from build123d import *

# Parameters (mm, degrees)
SKETCH2_R           = 4.5
BOSS_EXTRUDE1_DEPTH = 15
SKETCH4_R           = 4
CUT_EXTRUDE2_DEPTH  = 1.5
SKETCH5_R           = 3
CUT_EXTRUDE3_DEPTH  = 2.5
CUT_EXTRUDE4_DEPTH  = 6
SKETCH7_W           = 18
SKETCH7_H           = 2.5
BOSS_EXTRUDE2_DEPTH = 5


with BuildPart() as part:
    # Sketch2 → Boss-Extrude1 (new body)
    with BuildSketch(Plane(origin=(0, 0, 0), x_dir=(1, 0, 0), z_dir=(0, 1, 0))):
        Circle(SKETCH2_R)
    extrude(amount=BOSS_EXTRUDE1_DEPTH)

    # Sketch4 → Cut-Extrude2 (cut)
    with BuildSketch(Plane.XZ):
        with Locations((0, 0.009200476)):
            Circle(SKETCH4_R)
    extrude(amount=-CUT_EXTRUDE2_DEPTH, mode=Mode.SUBTRACT)

    # Sketch5 → Cut-Extrude3 (cut)
    with BuildSketch(Plane.XZ.offset(-1.5)):
        with Locations((0.006133651, -0.009200476)):
            Circle(SKETCH5_R)
    extrude(amount=-CUT_EXTRUDE3_DEPTH, mode=Mode.SUBTRACT)

    # Sketch6 → Cut-Extrude4 (cut)
    with BuildSketch(Plane.XZ.offset(-4)):
        with BuildLine():
            Line((-2.446188527, -1.739471433), (2.441510318, -1.739471433))
            ThreePointArc((2.441510318, -1.739471433), (2.997660896, 0.000528567), (2.441510318, 1.740528567))
            Line((2.441510318, 1.740528567), (-2.446188527, 1.740528567))
            ThreePointArc((-2.446188527, 1.740528567), (-3.002339104, 0.000528567), (-2.446188527, -1.739471433))
        make_face()
    extrude(amount=-CUT_EXTRUDE4_DEPTH, mode=Mode.SUBTRACT)

    # Sketch7 → Boss-Extrude2 (add)
    with BuildSketch(Plane(origin=(0, 15, 0), x_dir=(1, 0, 0), z_dir=(0, 1, 0))):
        Rectangle(SKETCH7_W, SKETCH7_H)
    extrude(amount=-BOSS_EXTRUDE2_DEPTH)


solid = part.part
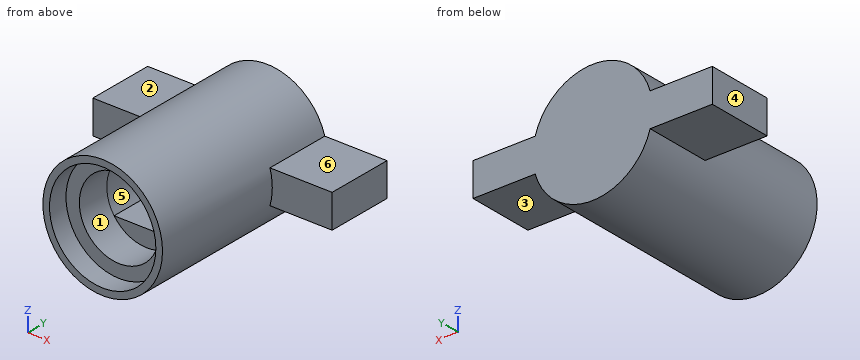
Work out the finished part from the listing and answer in its coordinate system (mm). Face numbers are marked on the shaded views. A direction names the side the tool comes from. Give positions to 0.01 mm unless a question says otherwise; leave off trailing zeros. Write each loop counter-clockwise with the first axis right and the second up, starting at its lowest first coordinate (ties: lowest second). Pieces come first, ordered by that corner, then holes. Notation, with made-up numbers: (73, 32) - (110, 32) arc R18 cw to (110, 54) - close; hole circle Ø9 at (28, 88.5). An arc over 180 degrees is marked (long way). One line per item, written item: value. Start each with the question number.
1. Consider probe 1 along Z at (x, y) = (0, 1.2); probe 2 along Y at (x, z) = (2.5, 3); probe 3 along Y at (x, z) = (5.25, 0). Determine where each line is inside the solid, lowest interval first.
2. Given pin 1 (2.5 mm diameter, centred on x = -2, z = 1.5, fed in from -Y); pin 2 (1.5 mm diameter, centred on x = 1, y = 7, fed in from -Z); pin 3 (5 mm diameter, centred on x = -6.5, y = 11.5, fed in from -Z), each flat-ended and moving along its own axis, determine where each tip first touches the part or whether it passes through.
3. Find section D-D (y = 1). Write down the section's boundary in (x, z), then the cut area to 3 significant figures.
4. For a pull along X with two mould halves and no side action, classify the marked faces 4, 5 and 6 as +X half, -X half, draft (parallel to the pull), parting line (faces both ways), or undercut.
5. Find section B-B (x = 0). Write down the section's boundary in (y, z), then the cut area to 3 significant figures.
6. For the marked faces 1, 2 and 3, determine the directions among +Z, -Z, +X, -X, +Y, -Y from which every point of the face is accessible in a straight line to the end or side of a thin tool.
7. Find section A-A (y = 10.75). Write down the section's boundary in (x, z), then the cut area to 3 significant figures.
8. Find section C-C (z = 2.25). Write down the section's boundary in (x, y).
Geometry results:
1. probe 1: -4.5 to -3.99, 4.01 to 4.5
1. probe 2: 1.5 to 15
1. probe 3: 10 to 15
2. pin 1: y = 1.5
2. pin 2: z = -4.49
2. pin 3: z = -2.06
3. outline: circle Ø9 at (0, 0); hole circle Ø8 at (0, 0.01)
3. area: 13.4 mm2
4. face 4: -X half
4. face 5: undercut
4. face 6: draft
5. outline: (0, -4.5) - (15, -4.5) - (15, 4.5) - (0, 4.5) - (0, 4.01) - (1.5, 4.01) - (1.5, 2.99) - (4, 2.99) - (4, 1.74) - (10, 1.74) - (10, -1.74) - (4, -1.74) - (4, -3.01) - (1.5, -3.01) - (1.5, -3.99) - (0, -3.99) - close
5. area: 87.1 mm2
6. face 1: -Y
6. face 2: +Z, -X, +Y, -Y
6. face 3: -Z, +X, +Y, -Y
7. outline: (-9, -1.25) - (-4.32, -1.25) arc R4.5 ccw to (4.32, -1.25) - (9, -1.25) - (9, 1.25) - (4.32, 1.25) arc R4.5 ccw to (-4.32, 1.25) - (-9, 1.25) - close
7. area: 86.4 mm2
8. outline: (-3.9, 0) - (-3.31, 0) - (-3.31, 1.5) - (-1.97, 1.5) - (-1.97, 4) - (1.98, 4) - (1.98, 1.5) - (3.31, 1.5) - (3.31, 0) - (3.9, 0) - (3.9, 15) - (-3.9, 15) - close
